Could you check a few things on this model? Use its own coordinates, in mm. Face numbers are marked on the shaded views. A direction names the side the tool comes from. Coordinates: 2 decimals unless noted, no trailing zeros. Order: outer loops, then holes, each group sorted by start corner. A loop starts at its lowest first (then second) coordinate and runs counter-clockwise, first axis right, second up. Notation, with made-up numbers: M 5,27.25 L 20,27.25 A10 cw 20,32.25 Z; hole C -34,-39.5 d10. An arc over 180 degrees is marked long. Write item = value, one per line. Start each with the question number.
from build123d import *

# Parameters (mm, degrees)
BASE_FLANGE1_DEPTH             = 20
EDGE_FLANGE1_STRIP_W           = 7
EDGE_FLANGE1_STRIP_H           = 1.25
EDGE_FLANGE1_STRIP_CUT_DEPTH   = 49
EDGE_FLANGE1_STRIP_2_W         = 7
EDGE_FLANGE1_STRIP_2_H         = 1.25
EDGE_FLANGE1_STRIP_CUT_2_DEPTH = 18
EDGE_FLANGE1_STRIP_3_W         = 7
EDGE_FLANGE1_STRIP_3_H         = 1.25
EDGE_FLANGE1_STRIP_CUT_3_DEPTH = 49
EDGE_FLANGE1_DEPTH             = 49
EDGE_FLANGE1_BEND_DEPTH        = 18
EDGE_FLANGE1_BEND_2_DEPTH      = 49
CUT_EXTRUDE1_DEPTH             = 47.952768821
CUT_EXTRUDE1_DEPTH_BACK        = 47.952768821
SKETCH15_R                     = 2.5
CUT_EXTRUDE2_DEPTH             = 54.61494661
CUT_EXTRUDE2_DEPTH_BACK        = 54.61494661
SKETCH16_R                     = 2.5
EDGE_FLANGE2_STRIP_W           = 7
EDGE_FLANGE2_STRIP_H           = 1.25
EDGE_FLANGE2_STRIP_CUT_DEPTH   = 38
EDGE_FLANGE2_RELIEF_W          = 7.625
EDGE_FLANGE2_RELIEF_H          = 0.625
EDGE_FLANGE2_RELIEF_CUT_DEPTH  = 1.25
EDGE_FLANGE2_DEPTH             = 38
CUT_EXTRUDE3_DEPTH             = 62.778333581
CUT_EXTRUDE3_DEPTH_BACK        = 1.25
SKETCH20_W                     = 25
SKETCH20_H                     = 13.5


# Sheet-metal steps are written as plain solids
with BuildPart() as part:
    # Sketch1 → Base-Flange1 (new body)
    with BuildSketch(Plane(origin=(0, 0, 0), x_dir=(1, 0, 0), z_dir=(0, 1, 0))):
        with BuildLine():
            Line((-10, -25), (-10, 24))
            ThreePointArc((-10, 24), (-9.707106781, 24.707106781), (-9, 25))
            Line((-9, 25), (9, 25))
            ThreePointArc((9, 25), (9.707106781, 24.707106781), (10, 24))
            Line((10, 24), (10, -25))
            Line((10, -25), (11.25, -25))
            Line((11.25, -25), (11.25, 24))
            ThreePointArc((11.25, 24), (10.590990258, 25.590990258), (9, 26.25))
            Line((9, 26.25), (-9, 26.25))
            ThreePointArc((-9, 26.25), (-10.590990258, 25.590990258), (-11.25, 24))
            Line((-11.25, 24), (-11.25, -25))
            Line((-11.25, -25), (-10, -25))
        make_face()
    extrude(amount=BASE_FLANGE1_DEPTH)

    # Edge-Flange1 strip (across the edge) → Edge-Flange1 strip cut (cut)
    with BuildSketch(Plane(origin=(-11.25, 0, -24), x_dir=(0, 1, 0), z_dir=(0, 0, 1))):
        with Locations((-1.25, -0.625)):
            Rectangle(EDGE_FLANGE1_STRIP_W, EDGE_FLANGE1_STRIP_H)
    extrude(amount=EDGE_FLANGE1_STRIP_CUT_DEPTH, mode=Mode.SUBTRACT)

    # Edge-Flange1 strip 2 (across the edge) → Edge-Flange1 strip cut 2 (cut)
    with BuildSketch(Plane(origin=(9, 0, -26.25), x_dir=(0, 1, 0), z_dir=(-1, 0, 0))):
        with Locations((-1.25, -0.625)):
            Rectangle(EDGE_FLANGE1_STRIP_2_W, EDGE_FLANGE1_STRIP_2_H)
    extrude(amount=EDGE_FLANGE1_STRIP_CUT_2_DEPTH, mode=Mode.SUBTRACT)

    # Edge-Flange1 strip 3 (across the edge) → Edge-Flange1 strip cut 3 (cut)
    with BuildSketch(Plane(origin=(11.25, 0, 25), x_dir=(0, 1, 0), z_dir=(0, 0, -1))):
        with Locations((-1.25, -0.625)):
            Rectangle(EDGE_FLANGE1_STRIP_3_W, EDGE_FLANGE1_STRIP_3_H)
    extrude(amount=EDGE_FLANGE1_STRIP_CUT_3_DEPTH, mode=Mode.SUBTRACT)

    # Edge-Flange1 section (across the edge) → Edge-Flange1 (add)
    with BuildSketch(Plane(origin=(-11.25, 0, -24), x_dir=(0, 1, 0), z_dir=(0, 0, 1))):
        with BuildLine():
            Line((0, 1), (0, 10.75))
            Line((0, 10.75), (1.25, 10.75))
            Line((1.25, 10.75), (1.25, 1))
            ThreePointArc((1.25, 1), (1.542893219, 0.292893219), (2.25, 0))
            Line((2.25, 0), (2.25, -1.25))
            ThreePointArc((2.25, -1.25), (0.659009742, -0.590990258), (0, 1))
        make_face()
    extrude(amount=EDGE_FLANGE1_DEPTH)

    # Edge-Flange1 section 2 (across the edge) → Edge-Flange1 bend (add)
    with BuildSketch(Plane(origin=(9, 0, -26.25), x_dir=(0, 1, 0), z_dir=(-1, 0, 0))):
        with BuildLine():
            Line((0, 1), (0, 10.75))
            Line((0, 10.75), (1.25, 10.75))
            Line((1.25, 10.75), (1.25, 1))
            ThreePointArc((1.25, 1), (1.542893219, 0.292893219), (2.25, 0))
            Line((2.25, 0), (2.25, -1.25))
            ThreePointArc((2.25, -1.25), (0.659009742, -0.590990258), (0, 1))
        make_face()
    extrude(amount=EDGE_FLANGE1_BEND_DEPTH)

    # Edge-Flange1 section 3 (across the edge) → Edge-Flange1 bend 2 (add)
    with BuildSketch(Plane(origin=(11.25, 0, 25), x_dir=(0, 1, 0), z_dir=(0, 0, -1))):
        with BuildLine():
            Line((0, 1), (0, 10.75))
            Line((0, 10.75), (1.25, 10.75))
            Line((1.25, 10.75), (1.25, 1))
            ThreePointArc((1.25, 1), (1.542893219, 0.292893219), (2.25, 0))
            Line((2.25, 0), (2.25, -1.25))
            ThreePointArc((2.25, -1.25), (0.659009742, -0.590990258), (0, 1))
        make_face()
    extrude(amount=EDGE_FLANGE1_BEND_2_DEPTH)

    # Sketch15 → Cut-Extrude1 (cut, two sides: drawn at the far end of the back side and taken through both)
    with BuildSketch(Plane(origin=(0, 1.25, 0), x_dir=(1, 0, 0), z_dir=(0, 1, 0)).offset(-CUT_EXTRUDE1_DEPTH_BACK)):
        with Locations(Location((17.125, -0.5, 0), (0, 0, 180))):
            Circle(SKETCH15_R)
        with Locations(Location((0, 32.125, 0), (0, 0, 180))):
            Circle(SKETCH15_R)
        with Locations(Location((-17.125, -0.5, 0), (0, 0, 180))):
            Circle(SKETCH15_R)
    extrude(amount=CUT_EXTRUDE1_DEPTH + CUT_EXTRUDE1_DEPTH_BACK, mode=Mode.SUBTRACT)

    # Sketch16 → Cut-Extrude2 (cut, two sides: drawn at the far end of the back side and taken through both)
    with BuildSketch(Plane(origin=(11.25, 0, 0), x_dir=(0, 0, -1), z_dir=(1, 0, 0)).offset(-CUT_EXTRUDE2_DEPTH_BACK)):
        with Locations((0, 11.125)):
            Circle(SKETCH16_R)
    extrude(amount=CUT_EXTRUDE2_DEPTH + CUT_EXTRUDE2_DEPTH_BACK, mode=Mode.SUBTRACT)

    # Edge-Flange2 strip (across the edge) → Edge-Flange2 strip cut (cut)
    with BuildSketch(Plane(origin=(22, 1.25, 14), x_dir=(-1, 0, 0), z_dir=(0, 0, -1))):
        with Locations((-2.5, -0.625)):
            Rectangle(EDGE_FLANGE2_STRIP_W, EDGE_FLANGE2_STRIP_H)
    extrude(amount=EDGE_FLANGE2_STRIP_CUT_DEPTH, mode=Mode.SUBTRACT)

    # Edge-Flange2 relief (on the sheet) → Edge-Flange2 relief cut (cut)
    with BuildSketch(Plane(origin=(21, 1.25, 14), x_dir=(-1, 0, 0), z_dir=(0, 1, 0))):
        with Locations((-3.1875, 0.3125)):
            Rectangle(EDGE_FLANGE2_RELIEF_W, EDGE_FLANGE2_RELIEF_H)
    extrude(amount=-EDGE_FLANGE2_RELIEF_CUT_DEPTH, mode=Mode.SUBTRACT)

    # Edge-Flange2 section (across the edge) → Edge-Flange2 (add)
    with BuildSketch(Plane(origin=(22, 1.25, 14), x_dir=(-1, 0, 0), z_dir=(0, 0, -1))):
        with BuildLine():
            Line((-1.25, 1), (-1.25, 16.75))
            Line((-1.25, 16.75), (0, 16.75))
            Line((0, 16.75), (0, 1))
            ThreePointArc((0, 1), (0.292893219, 0.292893219), (1, 0))
            Line((1, 0), (1, -1.25))
            ThreePointArc((1, -1.25), (-0.590990258, -0.590990258), (-1.25, 1))
        make_face()
    extrude(amount=EDGE_FLANGE2_DEPTH)

    # Sketch20 → Cut-Extrude3 (cut, two sides: drawn at the far end of the back side and taken through both)
    with BuildSketch(Plane(origin=(23.25, 0, 0), x_dir=(0, 0, -1), z_dir=(1, 0, 0)).offset(-CUT_EXTRUDE3_DEPTH_BACK)):
        with Locations((5.5, 11.25)):
            Rectangle(SKETCH20_W, SKETCH20_H)
    extrude(amount=CUT_EXTRUDE3_DEPTH + CUT_EXTRUDE3_DEPTH_BACK, mode=Mode.SUBTRACT)


solid = part.part
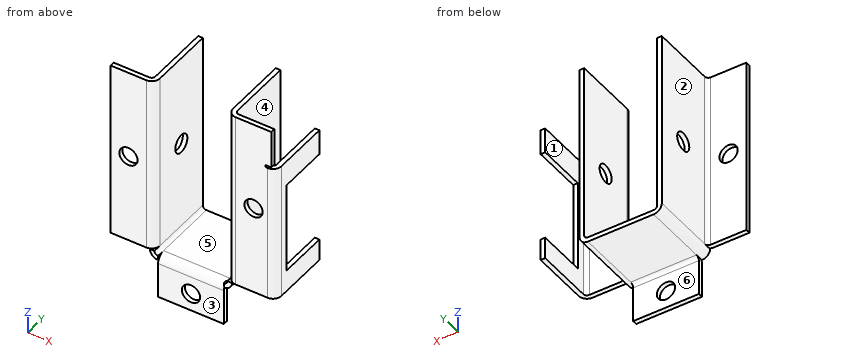
(1) Will these pins go through, and if not, where does the flat tip stop? P1, Ø5.5, axis at y = 11, z = 11, coming from the -X side; P2, Ø4, axis at x = -2, y = 16, coming from the +Z side; P3, Ø1.4, axis at x = 22.5, z = -20, coming from the +Y side.
(2) Imagine slicing it at D-D on y = 9.75. List the corners of the cut face in (x, z) for me, plus the area to 3 significant figures.
(3) Imagine slicing it at A-A on x = 0. List the corners of the cut face in (y, z) for me (3 decimals).
(4) Please list where these lines run through material, in increasing order: probe 1 along X at (y, z) = (16, 12.5); probe 2 along X at (y, z) = (14.5, 20); probe 3 along X at (y, z) = (0.7, 0.5) (3 decimals). Write a range as from..to.
(5) Thinking about a two-plate mould opening in X: for the marked faces 1, 2 and 3, which applies, released by +X, released by -X, zero draft, split by the parting line, or undercut?
(6) Imagine slicing it at C-C on x = 6. List the corners of the cut face in (y, z) for me.
(7) For the marked faces 4, 5 and 6, which set-ups out of +Z, -Z, +X, -X, +Y, -Y let a thin tool reach every point of the face, with its end or its side?
(8) Imagine slicing it at B-B on y = 17. List the corners of the cut face in (x, z) for me.
Response:
q1.P1 = -11.25
q1.P2 = -25
q1.P3 = 18
q2.outline = M -11.25,-24 A2.25 ccw -9,-26.25 L 9,-26.25 A2.25 ccw 11.25,-24 L 11.25,-2.09 L 10,-2.09 L 10,-24 A1 cw 9,-25 L -9,-25 A1 cw -10,-24 L -10,-2.09 L -11.25,-2.09 Z; M -11.25,2.09 L -10,2.09 L -10,25 L -11.25,25 Z; M 10,2.09 L 11.25,2.09 L 11.25,25 L 10,25 Z; M 22,-24 L 23.25,-24 L 23.25,-18 L 22,-18 Z; M 22,7 L 23.25,7 L 23.25,14 L 22,14 Z
q2.area = 157 mm2
q3.outline = M 0,-37 L 1.25,-37 L 1.25,-34.625 L 0,-34.625 Z; M 0,-29.625 L 1.25,-29.625 L 1.25,-27.25 A1 cw 2.25,-26.25 L 20,-26.25 L 20,-25 L 2.25,-25 A2.25 ccw 0,-27.25 Z
q4.probe_1 = -11.25..-10, 10..11.25, 22..23.25
q4.probe_2 = -11.25..-10, 10..11.25
q4.probe_3 = -22..-19.625, -14.625..-10.619, 10.619..14.625, 19.625..22.631
q5.face_1 = undercut
q5.face_2 = released by -X
q5.face_3 = zero draft
q6.outline = M 0,-37 L 1.25,-37 L 1.25,-27.25 A1 cw 2.25,-26.25 L 20,-26.25 L 20,-25 L 2.25,-25 A2.25 ccw 0,-27.25 Z
q7.face_4 = +Z, -Z, +Y
q7.face_5 = +Z, +Y, -Y
q7.face_6 = -Z, +X, -X, +Y
q8.outline = M -11.25,-24 A2.25 ccw -9,-26.25 L 9,-26.25 A2.25 ccw 11.25,-24 L 11.25,25 L 10,25 L 10,-24 A1 cw 9,-25 L -9,-25 A1 cw -10,-24 L -10,25 L -11.25,25 Z; M 22,-24 L 23.25,-24 L 23.25,-18 L 22,-18 Z; M 22,7 L 23.25,7 L 23.25,14 L 22,14 Z
